Answer from the drawing. Dimensions are ordinates in mm from the lowest x, y and z of the part. Round coordinates to 2 decimals unless told otherwise and drop trailing zeros. Loops run counter-clockwise (first coordinate to the right, second up) from the corner with the lowest first, then second, coordinate; pieces in that order, holes last. Notation, with made-up numbers: M -33.5,44.25 L -20.5,44.25 A9 cw -20.5,57.25 Z; hole C 28.5,-39.75 d8. An arc over 180 degrees is marked long. Answer as a JSON object with one key per item and string values.
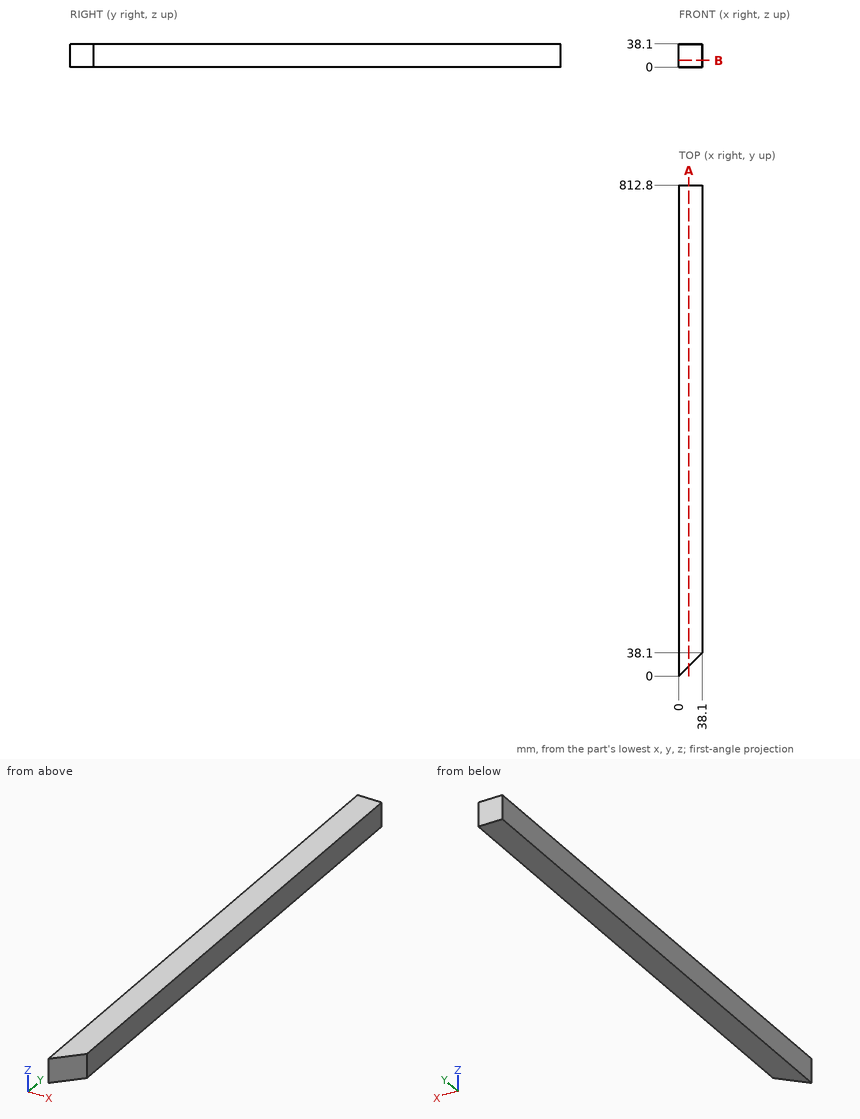
Item 1: The part is cut by section A-A (x = 16.5). Give the vertices of the cut face in (y, z).
Values follow:
{"outline": "M 16.5,0 L 812.8,0 L 812.8,38.1 L 16.5,38.1 Z"}
Item 2: The part is cut by section B-B (z = 11). Give the vertices of the cut face in (x, y), then the cut area to 3 significant figures.
Values follow:
{"outline": "M 0,0 L 38.1,38.1 L 38.1,812.8 L 0,812.8 Z", "area": "30,200 mm^2"}
Item 3: Straight lines are drawn through the part: line 1 (Y direction, x = 20.5, z = 7); line 2 (Y direction, x = 24.5, z = 31.5). For each, find the intervals that lie inside material, in ascending order.
Values follow:
{"line 1": "20.5 to 812.8", "line 2": "24.5 to 812.8"}
Item 4: A flat-ended cylindrical pin translates along its axis: P1, Ø12, axis at x = 4.5, y = 477.5, coming from the -Z side. Find the tip coordinate at first contact, or state that the pin passes through.
Values follow:
{"P1": "z = 0"}
